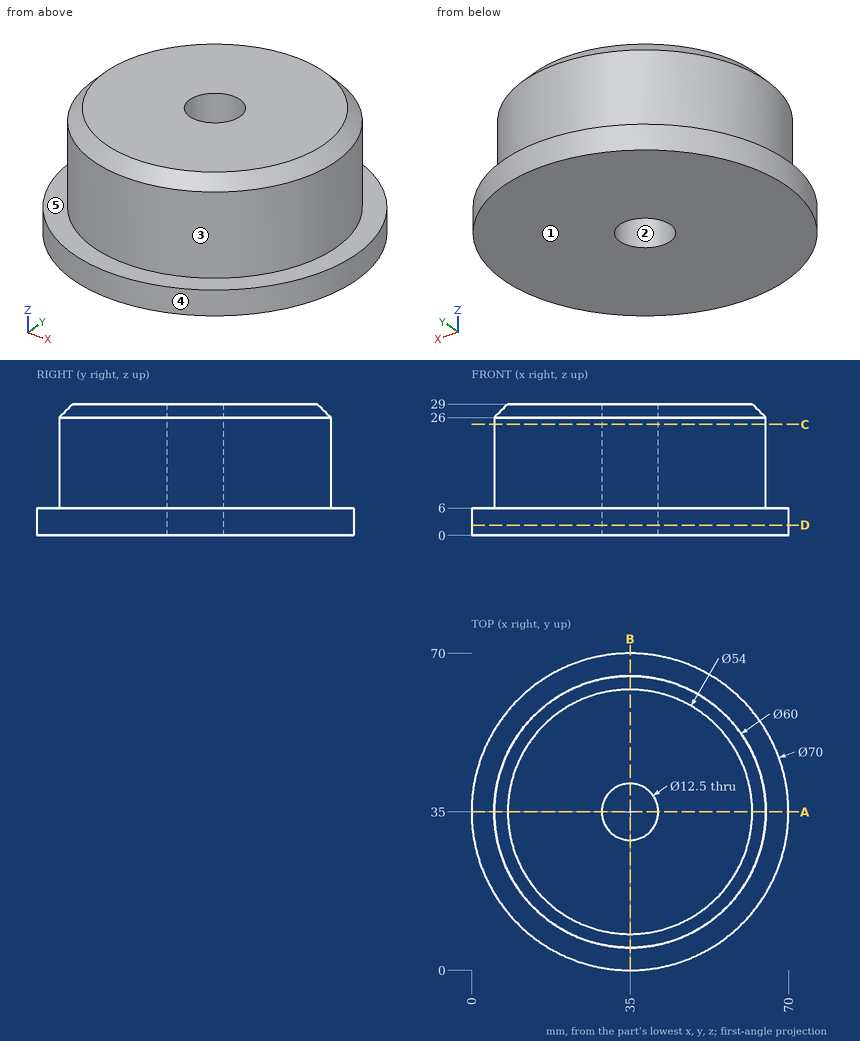
Could you check a few things on this drawing? It's one solid part, dimensions in mm from its lowest x, y, z. A direction names the side the tool comes from. Round coordinates to 2 decimals unless told otherwise and drop trailing zeros. Write each loop counter-clockwise with the first axis right and the second up, starting at its lowest first coordinate (ties: lowest second). Pieces come first, ordered by that corner, then holes. Notation, with made-up numbers: (35, 58) -> (44, 58) arc R15 ccw to (44, 73) -> close; hole circle Ø4 at (58, 40). An arc over 180 degrees is marked (long way). Use a Markdown table: item, result.
1. For pin 1 Ø10 at (y, z) = (35, 12.5) entering from -X; pin 2 Ø7.5 at (x, y) = (35, 35) entering from +Z; pin 3 Ø1.5 at (x, z) = (18.5, 10.5) entering from -Y; pin 4 Ø1.5 at (x, z) = (33.5, 5) entering from +Y, each with a flat end and sliding along its axis, tell me the tip position at first contact or that it passes through.
Answer key:
| item | result |
|---|---|
| pin 1 | stops at x = 5 |
| pin 2 | passes through |
| pin 3 | stops at y = 9.47 |
| pin 4 | stops at y = 69.99 |
2. If we section it at C-C (z = 24.5): List the corners of the cut face in (x, y) for me, then the cut area to 3 significant figures.
Answer key:
| item | result |
|---|---|
| outline | circle Ø60 at (35, 35); hole circle Ø12.5 at (35, 35) |
| area | 2,700 mm^2 |
3. If we section it at A-A (y = 35): List the corners of the cut face in (x, z) for me, then the cut area to 3 significant figures.
Answer key:
| item | result |
|---|---|
| outline | (0, 0) -> (28.75, 0) -> (28.75, 29) -> (8, 29) -> (5, 26) -> (5, 6) -> (0, 6) -> close; (41.25, 0) -> (70, 0) -> (70, 6) -> (65, 6) -> (65, 26) -> (62, 29) -> (41.25, 29) -> close |
| area | 1,430 mm^2 |
4. Which directions (+Z, -Z, +X, -X, +Y, -Y) give clear straight access to the entire face, cutting with the end or side of a thin tool? Please do the marked faces 4 and 5.
Answer key:
| item | result |
|---|---|
| face 4 | +Z, -Z |
| face 5 | +Z |
5. If we section it at D-D (z = 2.25): List the corners of the cut face in (x, y) for me, then the cut area to 3 significant figures.
Answer key:
| item | result |
|---|---|
| outline | circle Ø70 at (35, 35); hole circle Ø12.5 at (35, 35) |
| area | 3,730 mm^2 |
6. We'd pull the mould along X, two halves only. Please class the marked faces 1, 2 and 3: +X half, -X half, draft (parallel to the pull), parting line (faces both ways), or undercut.
Answer key:
| item | result |
|---|---|
| face 1 | draft |
| face 2 | undercut |
| face 3 | parting line |
7. Please list where these lines run through material, in increasing order: probe 1 along Y at (x, z) = (35, 7.5); probe 2 along Z at (x, y) = (4, 51); probe 3 along X at (y, z) = (50, 25.75).
Answer key:
| item | result |
|---|---|
| probe 1 | y = 5 to 28.75, 41.25 to 65 |
| probe 2 | z = 0 to 6 |
| probe 3 | x = 9.02 to 60.98 |
